from build123d import *

# Parameters (mm, degrees)
SKETCH1_W           = 19.812
SKETCH1_H           = 19.812
BOSS_EXTRUDE1_DEPTH = 9.652
BOSS_EXTRUDE1_TAPER = 6
FILLET1_R           = 1.27


with BuildPart() as part:
    # Sketch1 → Boss-Extrude1 (new body)
    with BuildSketch(Plane.XY):
        with Locations((9.906, -9.906)):
            Rectangle(SKETCH1_W, SKETCH1_H)
    extrude(amount=BOSS_EXTRUDE1_DEPTH, taper=BOSS_EXTRUDE1_TAPER)

    # Fillet1
    fillet1_edges = [part.edges().sort_by_distance(p)[0] for p in [
        (18.797533921, -9.906, 9.652),
        (9.906, -1.014466079, 9.652),
        (1.014466079, -9.906, 9.652),
        (0.507233039, -0.507233039, 4.826),
        (19.304766961, -0.507233039, 4.826),
        (19.304766961, -19.304766961, 4.826),
        (0.507233501, -19.304766499, 4.826004395),
        (9.906, -18.797533921, 9.652),
    ]]
    fillet(fillet1_edges, radius=FILLET1_R)


solid = part.part
The listing builds one solid part. Answer for the finished solid, in the listing's coordinates (mm). Give positions to 0.01 mm unless a question says otherwise; leave off trailing zeros. Loops run counter-clockwise (first coordinate to the right, second up) from the corner with the lowest first, then second, coordinate; pieces in that order, holes last.
Item 1: Find the intervals of material crossed by line 1 along Y through (x, z) = (11.75, 4); line 2 along Y through (x, z) = (7.25, 8.5); line 3 along X through (y, z) = (-10.25, 3), in increasing order.
Derived:
line 1: y = -19.39 to -0.42
line 2: y = -18.92 to -0.89
line 3: x = 0.32 to 19.5
Item 2: Each of these flat-tipped pins is pushed along its axis until it touches: pin 1 Ø1 at (x, z) = (9.5, 5) entering from -Y; pin 2 Ø5 at (y, z) = (-4.5, 5.5) entering from -X; pin 3 Ø3 at (y, z) = (-11.5, 5.5) entering from -X. Where does it stop, or does it pass through?
Derived:
pin 1: stops at y = -19.34
pin 2: stops at x = 0.32
pin 3: stops at x = 0.42
Item 3: A cutting plane is placed at B-B (y = -8.5). Give the vertices of the cut face in (x, z).
Derived:
outline: (0, 0) - (19.81, 0) - (18.92, 8.51) arc R1.27 ccw to (17.65, 9.65) - (2.16, 9.65) arc R1.27 ccw to (0.89, 8.51) - close
Item 4: A cutting plane is placed at A-A (x = 13.5). Give the vertices of the cut face in (y, z).
Derived:
outline: (-19.81, 0) - (0, 0) - (-0.89, 8.51) arc R1.27 ccw to (-2.16, 9.65) - (-17.65, 9.65) arc R1.27 ccw to (-18.92, 8.51) - close
